Could you check a few things on this model? Use its own coordinates, in mm. Face numbers are marked on the shaded views. Round coordinates to 2 decimals unless told otherwise and drop trailing zeros. Order: outer loops, then holes, each group sorted by start corner. A loop starts at its lowest first (then second) coordinate and runs counter-clockwise, first axis right, second up. Notation, with made-up numbers: (-25.75, -32) -> (1.25, -32) arc R24 ccw to (1.25, -16) -> close; hole circle Ø1 at (58, 85.5). An arc over 180 degrees is marked (long way). One line per question, with ' | ' between items.
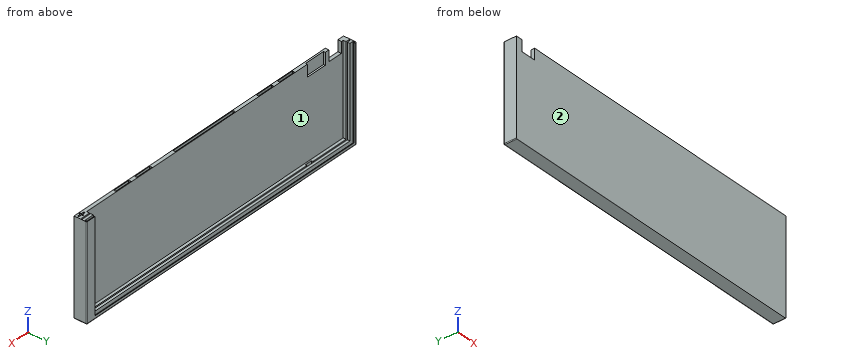
```python
from build123d import *

# Parameters (mm, degrees)
EXTRUDE_1_DEPTH     = 449.532
EXTRUDE_2_DEPTH     = 133.326
EXTRUDE_3_DEPTH     = 133.326
SKETCH_6_W          = 10
SKETCH_6_H          = 2
CUT_EXTRUDE_4_DEPTH = 5
SKETCH_7_W          = 15
SKETCH_7_H          = 2.5
CUT_EXTRUDE_5_DEPTH = 8.5
SKETCH_9_W          = 100
SKETCH_9_H          = 3
SKETCH_9_W_2        = 25
CUT_EXTRUDE_7_DEPTH = 30
SKETCH_10_W         = 21
SKETCH_10_H         = 5
CUT_EXTRUDE_8_DEPTH = 15.5
SKETCH_11_W         = 30
SKETCH_11_H         = 2.5
CUT_EXTRUDE_9_DEPTH = 17
FILLET_1_R          = 1
FILLET_2_R          = 1
FILLET_4_R          = 1


with BuildPart() as part:
    # 草图1 → 凸台-拉伸1 (new body)
    with BuildSketch(Plane(origin=(0, 0, 0), x_dir=(0, 0, -1), z_dir=(1, 0, 0))):
        Polygon((0, 0), (-4.2, 0), (-4.2, -1), (-1.5, -1), (-1.5, -3.55), (-6.5, -3.55), (-6.5, -7.25), (-1.5, -7.25), (-1.5, -8.9), (-6.5, -8.9), (-6.5, -12.9), (-133.326, -12.9), (-133.326, -17.9), (0, -17.9), align=None)
    extrude(amount=EXTRUDE_1_DEPTH)

    # 草图3 → 凸台-拉伸2 (add)
    with BuildSketch(Plane(origin=(0, 0, 0), x_dir=(-1, 0, 0), z_dir=(0, 0, -1))):
        Polygon((-449.532, 0), (-436.032, 0), (-436.032, -1), (-448.032, -1), (-448.032, -3.55), (-434.532, -3.55), (-434.532, -7.25), (-448.032, -7.25), (-448.032, -8.9), (-434.532, -8.9), (-434.532, -17.9), (-449.532, -17.9), align=None)
    extrude(amount=-EXTRUDE_2_DEPTH)

    # 草图4 → 凸台-拉伸3 (add)
    with BuildSketch(Plane(origin=(0, 0, 0), x_dir=(-1, 0, 0), z_dir=(0, 0, -1))):
        Polygon((0, 0), (-3.6, 0), (-3.6, -1), (-1.5, -1), (-1.5, -3.55), (-6.5, -3.55), (-6.5, -7.25), (-1.5, -7.25), (-1.5, -8.9), (-6.5, -8.9), (-6.5, -17.9), (0, -17.9), align=None)
    extrude(amount=-EXTRUDE_3_DEPTH)

    # 草图6 → 切除-拉伸4 (cut)
    with BuildSketch(Plane.XY.offset(6.5)):
        with Locations((67, -9.9)):
            Rectangle(SKETCH_6_W, SKETCH_6_H)
    extrude(amount=-CUT_EXTRUDE_4_DEPTH, mode=Mode.SUBTRACT)

    # 草图7 → 切除-拉伸5 (cut)
    with BuildSketch(Plane.ZY.offset(-434.532)):
        with Locations((23.5, -10.15)):
            Rectangle(SKETCH_7_W, SKETCH_7_H)
    extrude(amount=-CUT_EXTRUDE_5_DEPTH, mode=Mode.SUBTRACT)

    # 草图9 → 切除-拉伸7 (cut)
    with BuildSketch(Plane.XY.offset(133.326)):
        with Locations((235.515, -15.4)):
            Rectangle(SKETCH_9_W, SKETCH_9_H)
        with Locations((99, -15.4)):
            Rectangle(SKETCH_9_W_2, SKETCH_9_H)
        with Locations((337.032, -15.4)):
            Rectangle(SKETCH_9_W_2, SKETCH_9_H)
        with Locations((134, -15.4)):
            Rectangle(SKETCH_9_W_2, SKETCH_9_H)
        with Locations((372.032, -15.4)):
            Rectangle(SKETCH_9_W_2, SKETCH_9_H)
        Polygon((437.032, -12.9), (437.032, -14.9), (441.032, -14.9), (441.032, -16.9), (443.032, -16.9), (443.032, -14.9), (447.032, -14.9), (447.032, -12.9), (443.032, -12.9), (443.032, -10.9), (441.032, -10.9), (441.032, -12.9), align=None)
    extrude(amount=-CUT_EXTRUDE_7_DEPTH, mode=Mode.SUBTRACT)

    # 草图10 → 切除-拉伸8 (cut)
    with BuildSketch(Plane.XY.offset(133.326)):
        with Locations((20.053070751, -15.4)):
            Rectangle(SKETCH_10_W, SKETCH_10_H)
    extrude(amount=-CUT_EXTRUDE_8_DEPTH, mode=Mode.SUBTRACT)

    # 草图11 → 切除-拉伸9 (cut)
    with BuildSketch(Plane.XY.offset(133.326)):
        with Locations((51.5, -14.15)):
            Rectangle(SKETCH_11_W, SKETCH_11_H)
    extrude(amount=-CUT_EXTRUDE_9_DEPTH, mode=Mode.SUBTRACT)

    # 圆角1
    fillet_1_edges = [part.edges().sort_by_distance(p)[0] for p in [
        (0, 0, 66.663),
    ]]
    fillet(fillet_1_edges, radius=FILLET_1_R)

    # 圆角2
    fillet_2_edges = [part.edges().sort_by_distance(p)[0] for p in [
        (0, -9.45, 0),
        (225.266, 0, 0),
        (0.292893219, -0.292893219, 0),
    ]]
    fillet(fillet_2_edges, radius=FILLET_2_R)

    # 圆角4
    fillet_4_edges = [part.edges().sort_by_distance(p)[0] for p in [
        (449.532, 0, 67.163),
        (449.532, -0.292893219, 0.292893219),
        (449.532, -9.45, 0),
    ]]
    fillet(fillet_4_edges, radius=FILLET_4_R)


solid = part.part
```
1. I want a section at A-A on x = 343. List the corners of the cut face in (y, z) for me, and give its area (3 significant figures).
From the geometry:
outline: (-17.9, 0) -> (-1, 0) arc R1 ccw to (0, 1) -> (0, 4.2) -> (-1, 4.2) -> (-1, 1.5) -> (-3.55, 1.5) -> (-3.55, 6.5) -> (-7.25, 6.5) -> (-7.25, 1.5) -> (-8.9, 1.5) -> (-8.9, 6.5) -> (-12.9, 6.5) -> (-12.9, 133.33) -> (-13.9, 133.33) -> (-13.9, 103.33) -> (-16.9, 103.33) -> (-16.9, 133.33) -> (-17.9, 133.33) -> close | area: 637 mm²
2. I'm going to push flat-ended pins straight in: pin 1 (1 mm diameter, centred on x = 103, z = 51.5, fed in from +Y); pin 2 (5 mm diameter, centred on x = 241, y = -5, fed in from +Z). Where does each tip first touch, or does it pass through?
From the geometry:
pin 1: stops at y = -12.9 | pin 2: stops at z = 6.5
3. I want a section at B-B on z = 125. Count the separate pieces of the cut face and the enclosed holes in it, and give its area (3 significant figures).
From the geometry:
separate pieces: 2 | enclosed holes: 6 | area: 1,630 mm²
4. I want a section at C-C on z = 38.5. List the corners of the cut face in (x, y) for me.
From the geometry:
outline: (0, -17.9) -> (449.53, -17.9) -> (449.53, -1) arc R1 ccw to (448.53, 0) -> (436.03, 0) -> (436.03, -1) -> (448.03, -1) -> (448.03, -3.55) -> (434.53, -3.55) -> (434.53, -7.25) -> (448.03, -7.25) -> (448.03, -8.9) -> (434.53, -8.9) -> (434.53, -12.9) -> (6.5, -12.9) -> (6.5, -8.9) -> (1.5, -8.9) -> (1.5, -7.25) -> (6.5, -7.25) -> (6.5, -3.55) -> (1.5, -3.55) -> (1.5, -1) -> (3.6, -1) -> (3.6, 0) -> (1, 0) arc R1 ccw to (0, -1) -> close
5. If we mould it in two halves opening along X, with no side actions, what happens to the marked faces 1 and 2? For each: pulls with the +X half, pulls with the -X half, needs draft (parallel to the pull), parting line crosses it, or undercut.
From the geometry:
face 1: undercut | face 2: needs draft
6. I need wall thicknesses on probe 1 along X at (y, z) = (-11.25, 115); probe 2 along X at (y, z) = (-1.5, 119.5); probe 3 along X at (y, z) = (-12.75, 78). Which ranges of each line are inside material? Lowest first, please.
From the geometry:
probe 1: x = 0 to 6.5, 434.53 to 441.03, 443.03 to 449.53 | probe 2: x = 0 to 1.5, 448.03 to 449.53 | probe 3: x = 0 to 6.5, 434.53 to 449.53
